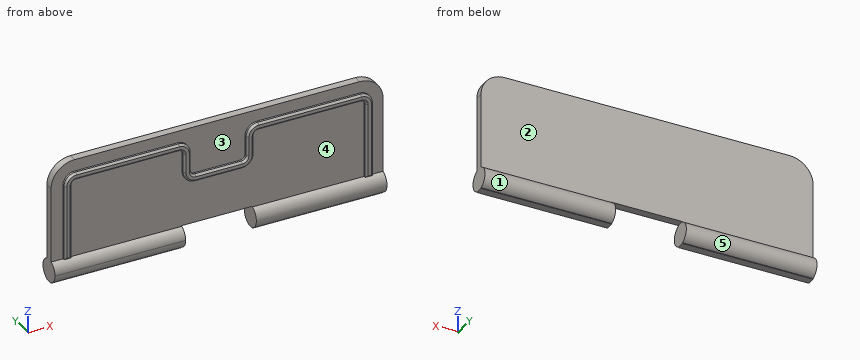
```python
from build123d import *

# Parameters (mm, degrees)
F0_W     = 33.259
F0_H     = 5.75
F1_DEPTH = 2
F3_DEPTH = 33.259
F6_DEPTH = 33.259
F4_W     = 1.8128321722
F4_H     = 19.1795176684
F4_W_2   = 26.160747505
F4_H_2   = 1.8128321722
F4_H_3   = 4.8250346239
F4_W_3   = 5.911082495
F4_H_4   = 1.81283
F7_DEPTH = 1
F8_SIZE  = 0.5


# Not quite as in the source:
# - ends of sketch curves that miss each other by under 0.0002 mm in the source are joined
# - a pattern or mirror of a feature is missing from the dataset's text; its kind, count and spacing are read off the source's solid


with BuildPart() as f1:
    # F0 (on Front) → F1 (new body)
    with BuildSketch(Plane.XZ):
        with BuildLine():
            Line((36.259, 12.5), (-36.259, 12.5))
            ThreePointArc((-36.259, 12.5), (-40.5016406871, 10.7426406871), (-42.259, 6.5))
            Line((-42.259, 6.5), (-42.259, -12.5))
            Line((-42.259, -12.5), (-9, -12.5))
            Line((-9, -12.5), (-3.6677482234, -11.0712274426))
            Line((-3.6677482234, -11.0712274426), (3.6677482234, -11.0712274426))
            Line((3.6677482234, -11.0712274426), (9, -12.5))
            Line((9, -12.5), (42.259, -12.5))
            Line((42.259, -12.5), (42.259, 6.5))
            ThreePointArc((42.259, 6.5), (40.5016406871, 10.7426406871), (36.259, 12.5))
        make_face()
        with Locations((-25.6295, -15.375)):
            Rectangle(F0_W, F0_H)
        with Locations((25.6295, -15.375)):
            Rectangle(F0_W, F0_H)
        Polygon((-3.6677482234, -11.0712274426), (-9, -12.5), (9, -12.5), (3.6677482234, -11.0712274426), align=None)
    extrude(amount=F1_DEPTH)

    # F2 (on face) → F3 (join, through all)
    with BuildSketch(Plane(origin=(-42.259, 0, 0), x_dir=(0, -1, 0), z_dir=(-1, 0, 0))):
        with BuildLine():
            ThreePointArc((3.875, -15.375), (3.3601509486, -13.7332593079), (2, -12.6795176684))
            Line((2, -12.6795176684), (2, -18.0704823316))
            ThreePointArc((2, -18.0704823316), (3.3601509486, -17.0167406921), (3.875, -15.375))
        make_face()
        with BuildLine():
            Line((2, -18.0704823316), (2, -12.6795176684))
            ThreePointArc((2, -12.6795176684), (-1.875, -15.375), (2, -18.0704823316))
        make_face()
    extrude(amount=-F3_DEPTH)

    # F5 (on face) → F6 (join, through all)
    with BuildSketch(Plane.YZ.offset(42.259)):
        with BuildLine():
            ThreePointArc((0, -18.0704823316), (1.875, -15.375), (0, -12.6795176684))
            Line((0, -12.6795176684), (0, -12.5))
            Line((0, -12.5), (-2, -12.5))
            Line((-2, -12.5), (-2, -12.6795176684))
            ThreePointArc((-2, -12.6795176684), (-3.875, -15.375), (-2, -18.0704823316))
            Line((-2, -18.0704823316), (-2, -18.25))
            Line((-2, -18.25), (0, -18.25))
            Line((0, -18.25), (0, -18.0704823316))
        make_face()
    extrude(amount=-F6_DEPTH)

    # F4 (on face) → F7 (join)
    with BuildSketch(Plane.XZ.offset(2)):
        with Locations((-38.3525839139, -3.0897588342)):
            Rectangle(F4_W, F4_H)
        with BuildLine():
            ThreePointArc((-36.259, 9.5), (-38.3803203436, 8.6213203436), (-39.259, 6.5))
            Line((-39.259, 6.5), (-37.4461678278, 6.5))
            ThreePointArc((-37.4461678278, 6.5), (-37.0984544214, 7.3394544214), (-36.259, 7.6871678278))
            Line((-36.259, 7.6871678278), (-36.259, 9.5))
        make_face()
        with Locations((-23.1786262475, 8.5935839139)):
            Rectangle(F4_W_2, F4_H_2)
        with BuildLine():
            ThreePointArc((-7.098252495, 6.5), (-7.9769321514, 8.6213203436), (-10.098252495, 9.5))
            Line((-10.098252495, 9.5), (-10.098252495, 7.6871678278))
            ThreePointArc((-10.098252495, 7.6871678278), (-9.2587980736, 7.3394544214), (-8.9110846672, 6.5))
            Line((-8.9110846672, 6.5), (-7.098252495, 6.5))
        make_face()
        with Locations((-8.0046685811, 4.087482688)):
            Rectangle(F4_W, F4_H_3)
        with Locations((-2.9555412475, -0.4186196239)):
            Rectangle(F4_W_3, F4_H_4)
        with BuildLine():
            ThreePointArc((-5.911082495, 0.4877953761), (-6.7505384524, 0.8355094187), (-7.098252495, 1.6749653761))
            Line((-7.098252495, 1.6749653761), (-8.9110846672, 1.6749653761))
            ThreePointArc((-8.9110846672, 1.6749653761), (-8.0324028386, -0.4463549675), (-5.911082495, -1.3250346239))
            Line((-5.911082495, -1.3250346239), (-5.911082495, 0.4877953761))
        make_face()
    f7 = extrude(amount=F7_DEPTH)

    # F7_copies: F7 across plane
    add(f7.mirror(Plane(origin=(0, 0, 0), x_dir=(0, 0, 1), z_dir=(1, 0, 0))))

    # F8
    f8_edges = [f1.edges().sort_by_distance(p)[0] for p in [
        (39.259, -3, -3.089759),
        (38.352584, -3, -12.679518),
        (37.446168, -3, -3.089759),
        (37.098454, -3, 7.339454),
        (23.178626, -3, 7.687168),
        (9.258798, -3, 7.339454),
        (8.911085, -3, 4.087483),
        (8.032403, -3, -0.446355),
        (0, -3, -1.325035),
        (-8.032403, -3, -0.446355),
        (-8.911085, -3, 4.087483),
        (-9.258798, -3, 7.339454),
        (-23.178626, -3, 7.687168),
        (-37.098454, -3, 7.339454),
        (-37.446168, -3, -3.089759),
        (-38.352584, -3, -12.679518),
        (-39.259, -3, -3.089759),
        (-38.38032, -3, 8.62132),
        (-23.178626, -3, 9.5),
        (-7.976932, -3, 8.62132),
        (-7.098252, -3, 4.087483),
        (-6.750538, -3, 0.835509),
        (0, -3, 0.487795),
        (6.750538, -3, 0.835509),
        (7.098252, -3, 4.087483),
        (7.976932, -3, 8.62132),
        (23.178626, -3, 9.5),
        (38.38032, -3, 8.62132),
    ]]
    chamfer(f8_edges, length=F8_SIZE)


solid = f1.part
```
Input: part model. Units: mm. Frame: model coordinates. Face numbers are marked on the shaded views. A direction names the side the tool comes from. Round coordinates to 2 decimals unless told otherwise and drop trailing zeros. Order: outer loops, then holes, each group sorted by start corner. A loop starts at its lowest first (then second) coordinate and runs counter-clockwise, first axis right, second up. Notation, with made-up numbers: (51.5, 41.5) - (97.5, 41.5) arc R28 ccw to (97.5, 78.5) - close; hole circle Ø1 at (-4, -36.5). An arc over 180 degrees is marked (long way). Answer in a Markdown table with one row per item.
Item 1: Mould query, pull axis X, two halves, no side actions, for the marked faces 4 and 5. Classes: released by +X, released by -X, zero draft, split by the parting line, or undercut.
Model answer:
| item | result |
|---|---|
| face 4 | undercut |
| face 5 | zero draft |
Item 2: Line query: line 1 (X direction, y = -2.25, z = 0); line 2 (X direction, y = 1.45, z = -15); line 3 (Y direction, x = -36.5, z = -9). Output: solid intervals per line, ascending.
Model answer:
| item | result |
|---|---|
| line 1 | x = -39.26 to -37.45, -8.4 to 8.4, 37.45 to 39.26 |
| line 2 | x = -42.26 to -9, 9 to 42.26 |
| line 3 | y = -2 to 0 |
Item 3: Section query D-D (z = 2.5). Return the cut outline in (x, y), then the cut area to 3 significant figures.
Model answer:
| item | result |
|---|---|
| outline | (-42.26, -2) - (-39.26, -2) - (-39.26, -2.5) - (-38.76, -3) - (-37.95, -3) - (-37.45, -2.5) - (-37.45, -2) - (-8.91, -2) - (-8.91, -2.5) - (-8.41, -3) - (-7.6, -3) - (-7.1, -2.5) - (-7.1, -2) - (7.1, -2) - (7.1, -2.5) - (7.6, -3) - (8.41, -3) - (8.91, -2.5) - (8.91, -2) - (37.45, -2) - (37.45, -2.5) - (37.95, -3) - (38.76, -3) - (39.26, -2.5) - (39.26, -2) - (42.26, -2) - (42.26, 0) - (-42.26, 0) - close |
| area | 175 mm² |
Item 4: Section query A-A (y = -1). Return the cut outline in (x, z), then the cut area to 3 significant figures.
Model answer:
| item | result |
|---|---|
| outline | (-42.26, -18.25) - (-9, -18.25) - (-9, -12.5) - (9, -12.5) - (9, -18.25) - (42.26, -18.25) - (42.26, 6.5) arc R6 ccw to (36.26, 12.5) - (-36.26, 12.5) arc R6 ccw to (-42.26, 6.5) - close |
| area | 2,480 mm² |
Item 5: Reachability of the marked faces 1, 2 and 3 from +Z, -Z, +X, -X, +Y, -Y: full face, straight path, thin tool, end or side. Return the list, or none.
Model answer:
| item | result |
|---|---|
| face 1 | +X, -X, +Y |
| face 2 | +Z, +X, -X, +Y |
| face 3 | +Z, -Y |
Item 6: Pin query (flat end, axial travel): pin 1 (8 mm diameter, centred on x = -14, z = 6, fed in from +Y); pin 2 (1 mm diameter, centred on x = -3, y = -1, fed in from -Z); pin 3 (10 mm diameter, centred on x = 17.5, z = -12, fed in from +Y) (3 decimals); pin 4 (10.5 mm diameter, centred on x = -14.5, z = 0, fed in from -Y). Return the tip coordinate at first contact, or that it passes through.
Model answer:
| item | result |
|---|---|
| pin 1 | stops at y = 0 |
| pin 2 | stops at z = -12.5 |
| pin 3 | stops at y = 1.875 |
| pin 4 | stops at y = -2 |
Item 7: Section query B-B (z = -4). Return the cut outline in (x, y), then the cut area to 3 significant figures.
Model answer:
| item | result |
|---|---|
| outline | (-42.26, -2) - (-39.26, -2) - (-39.26, -2.5) - (-38.76, -3) - (-37.95, -3) - (-37.45, -2.5) - (-37.45, -2) - (37.45, -2) - (37.45, -2.5) - (37.95, -3) - (38.76, -3) - (39.26, -2.5) - (39.26, -2) - (42.26, -2) - (42.26, 0) - (-42.26, 0) - close |
| area | 172 mm² |
Item 8: Section query C-C (x = -26.5). Return the cut outline in (y, z) (3 decimals), then the cut area to 3 significant figures.
Model answer:
| item | result |
|---|---|
| outline | (-3, 8.187) - (-2.5, 7.687) - (-2, 7.687) - (-2, -12.68) arc R2.875 ccw to (-2, -18.07) - (-2, -18.25) - (0, -18.25) - (0, -18.07) arc R2.875 ccw to (0, -12.68) - (0, 12.5) - (-2, 12.5) - (-2, 9.5) - (-2.5, 9.5) - (-3, 9) - close |
| area | 77.8 mm² |
